from build123d import *

# Parameters (mm, degrees)
SKETCH1_R               = 87
BOSS_EXTRUDE1_DEPTH     = 87.5
SKETCH2_R               = 9.4488
CUT_EXTRUDE1_DEPTH      = 1
CUT_EXTRUDE1_DEPTH_BACK = 176
SKETCH3_R               = 69.5
CUT_EXTRUDE2_DEPTH      = 10
SKETCH7_R               = 7.5
CUT_EXTRUDE3_DEPTH      = 166
CIRPATTERN1_COUNT       = 5


with BuildPart() as part:
    # Sketch1 → Boss-Extrude1 (new body, symmetric)
    with BuildSketch(Plane.XY):
        Circle(SKETCH1_R)
    extrude(amount=BOSS_EXTRUDE1_DEPTH, both=True)

    # Sketch2 → Cut-Extrude1 (cut, two sides)
    with BuildSketch(Plane.XY.offset(87.5)) as cut_extrude1_sk:
        Circle(SKETCH2_R)
    extrude(amount=CUT_EXTRUDE1_DEPTH, mode=Mode.SUBTRACT)
    extrude(cut_extrude1_sk.sketch, amount=-CUT_EXTRUDE1_DEPTH_BACK, mode=Mode.SUBTRACT)

    # Sketch3 → Cut-Extrude2 (cut)
    with BuildSketch(Plane.XY.offset(87.5)):
        Circle(SKETCH3_R)
    cut_extrude2 = extrude(amount=-CUT_EXTRUDE2_DEPTH, mode=Mode.SUBTRACT)

    # Mirror1: Cut-Extrude2 across plane
    add(cut_extrude2.mirror(Plane.XY), mode=Mode.SUBTRACT)

    # Sketch5 → Cut-Revolve1 (revolve, cut)
    with BuildSketch(Plane(origin=(0, 0, 0), x_dir=(1, 0, 0), z_dir=(0, 1, 0))):
        Polygon((87, 84.5), (81, 81.035898385), (81, -81.035898385), (87, -84.5), align=None)
    revolve(axis=Axis((0, 0, 0), (0, 0, -1)), mode=Mode.SUBTRACT)

    # Sketch7 → Cut-Extrude3 (cut, through all)
    with BuildSketch(Plane.XY.offset(77.5)):
        with Locations((0, 45)):
            Circle(SKETCH7_R)
    cut_extrude3 = extrude(amount=-CUT_EXTRUDE3_DEPTH, mode=Mode.SUBTRACT)

    # CirPattern1: Cut-Extrude3 ×5 about axis
    cirpattern1_axis = Axis((0, 0, 0), (0, 0, 1))
    for i in range(1, CIRPATTERN1_COUNT):
        add(cut_extrude3.rotate(cirpattern1_axis, i * 360 / CIRPATTERN1_COUNT), mode=Mode.SUBTRACT)


solid = part.part
Verification items for the finished model (mm, model axes). A direction names the side the tool comes from. Round coordinates to 2 decimals unless told otherwise and drop trailing zeros. Write each loop counter-clockwise with the first axis right and the second up, starting at its lowest first coordinate (ties: lowest second). Pieces come first, ordered by that corner, then holes.
(1) Material ranges on line 1 (Y direction, x = 0, z = -42); line 2 (X direction, y = -31.5, z = 62); line 3 (Y direction, x = 0, z = -80), recorded low to high.
Returned:
line 1: y = -81 to -9.45, 9.45 to 37.5, 52.5 to 81
line 2: x = -74.62 to -32.12, -20.78 to 20.78, 32.12 to 74.62
line 3: y = -81 to -69.5, 69.5 to 81
(2) Section check C-C (z = 72). Enter the section's corners in (x, y), plus the area to 3 significant figures.
Returned:
outline: circle Ø162 at (0, 0); hole circle Ø15 at (-42.8, 13.91); hole circle Ø15 at (-26.45, -36.41); hole circle Ø18.9 at (0, 0); hole circle Ø15 at (0, 45); hole circle Ø15 at (26.45, -36.41); hole circle Ø15 at (42.8, 13.91)
area: 19,400 mm2
(3) Access from +Z, -Z, +X, -X, +Y, -Y to the whole of each face (thin tool, end or side, straight path). Record for faces 1 (the cylindrical face through (37.363, 58.603, -82.57)), 2 (the flat face through (-1, -14, 77.5)), 3 (the cylindrical face through (43.545, -68.3, 1.135)), 4 (the cylindrical face through (-11.33, 86.26, 86.02)).
Returned:
face 1: -Z
face 2: +Z
face 3: none
face 4: +Z, -Z
(4) Depth check by flat-ended pin: pin 1 Ø24 at (x, y) = (26.45, -36.41) entering from +Z; pin 2 Ø1 at (y, z) = (63, 26) entering from -X; pin 3 Ø4 at (y, z) = (64.5, -42.5) entering from +X. Enter the tip coordinate at first touch or a pass-through.
Returned:
pin 1: stops at z = 77.5
pin 2: stops at x = -51.52
pin 3: stops at x = 51.52
(5) Mould release check, pull along Z, two halves, no side actions. Record for faces 5 (the flat face through (-58.4, -38.3, -87.5)), 6 (the conical face through (77.618, -24.443, 81.253)), 7 (the cylindrical face through (37.363, 58.603, 82.57)), 8 (the flat face through (-58.4, -38.3, 87.5)): pulls with the +Z half, pulls with the -Z half, needs draft (parallel to the pull), parting line crosses it, or undercut.
Returned:
face 5: pulls with the -Z half
face 6: undercut
face 7: needs draft
face 8: pulls with the +Z half
(6) Section check B-B (y = 0). Enter the section's corners in (x, z), plus the area to 3 significant figures.
Returned:
outline: (-87, -87.5) - (-69.5, -87.5) - (-69.5, -77.5) - (-9.45, -77.5) - (-9.45, 77.5) - (-69.5, 77.5) - (-69.5, 87.5) - (-87, 87.5) - (-87, 84.5) - (-81, 81.04) - (-81, -81.04) - (-87, -84.5) - close; (9.45, -77.5) - (69.5, -77.5) - (69.5, -87.5) - (87, -87.5) - (87, -84.5) - (81, -81.04) - (81, 81.04) - (87, 84.5) - (87, 87.5) - (69.5, 87.5) - (69.5, 77.5) - (9.45, 77.5) - close
area: 22,800 mm2
(7) Section check A-A (x = 0). Enter the section's corners in (y, z), plus the area to 3 significant figures.
Returned:
outline: (-87, -87.5) - (-69.5, -87.5) - (-69.5, -77.5) - (-9.45, -77.5) - (-9.45, 77.5) - (-69.5, 77.5) - (-69.5, 87.5) - (-87, 87.5) - (-87, 84.5) - (-81, 81.04) - (-81, -81.04) - (-87, -84.5) - close; (9.45, -77.5) - (37.5, -77.5) - (37.5, 77.5) - (9.45, 77.5) - close; (52.5, -77.5) - (69.5, -77.5) - (69.5, -87.5) - (87, -87.5) - (87, -84.5) - (81, -81.04) - (81, 81.04) - (87, 84.5) - (87, 87.5) - (69.5, 87.5) - (69.5, 77.5) - (52.5, 77.5) - close
area: 20,400 mm2
